Geometry: final body of the model. Coordinates: model frame, mm. A direction names the side the tool comes from. Round coordinates to 2 decimals unless told otherwise and drop trailing zeros. Loops run counter-clockwise (first coordinate to the right, second up) from the corner with the lowest first, then second, coordinate; pieces in that order, holes last. Notation, with made-up numbers: (49.25, 33.25) -> (102.25, 33.25) arc R21 ccw to (102.25, 67.25) -> close; hole circle Ø2 at (56, 63). An arc over 180 degrees is marked (long way). Answer in a Markdown table with one row per item.
```python
from build123d import *

# Parameters (mm, degrees)
SKETCH1_W               = 3.96875
SKETCH1_H               = 3.96875
BOSS_EXTRUDE1_DEPTH     = 12.5
SKETCH2_W               = 3.175
SKETCH2_H               = 3.175
CUT_EXTRUDE1_DEPTH      = 26.157016681
CUT_EXTRUDE2_DEPTH      = 13.811147032
CUT_EXTRUDE2_DEPTH_BACK = 13.811147032
SKETCH3_R               = 0.79375


with BuildPart() as part:
    # Sketch1 → Boss-Extrude1 (new, symmetric)
    with BuildSketch(Plane(origin=(0, 0, 0), x_dir=(1, 0, 0), z_dir=(0, 1, 0))):
        Rectangle(SKETCH1_W, SKETCH1_H)
    extrude(amount=BOSS_EXTRUDE1_DEPTH, both=True)

    # Sketch2 → Cut-Extrude1 (cut, through all)
    with BuildSketch(Plane(origin=(0, 12.5, 0), x_dir=(1, 0, 0), z_dir=(0, 1, 0))):
        Rectangle(SKETCH2_W, SKETCH2_H)
    extrude(amount=-CUT_EXTRUDE1_DEPTH, mode=Mode.SUBTRACT)

    # Sketch3 → Cut-Extrude2 (cut, two sides: drawn at the far end of the back side and taken through both)
    with BuildSketch(Plane.XY.offset(-CUT_EXTRUDE2_DEPTH_BACK)):
        with Locations((0, -10)):
            Circle(SKETCH3_R)
    extrude(amount=CUT_EXTRUDE2_DEPTH + CUT_EXTRUDE2_DEPTH_BACK, mode=Mode.SUBTRACT)


solid = part.part
```
Item 1: Cut plane A-A (x = 0). Output: boundary loops of the cut face in (y, z), then the cut area to 3 significant figures.
Answer:
| item | result |
|---|---|
| outline | (-12.5, -1.98) -> (-10.79, -1.98) -> (-10.79, -1.59) -> (-12.5, -1.59) -> close; (-12.5, 1.59) -> (-10.79, 1.59) -> (-10.79, 1.98) -> (-12.5, 1.98) -> close; (-9.21, -1.98) -> (12.5, -1.98) -> (12.5, -1.59) -> (-9.21, -1.59) -> close; (-9.21, 1.59) -> (12.5, 1.59) -> (12.5, 1.98) -> (-9.21, 1.98) -> close |
| area | 18.6 mm² |
Item 2: Reachability of faces 4 (the face through (-1.984, 0, 0)), 5 (the face through (0, 0, -1.588)) from +Z, -Z, +X, -X, +Y, -Y: full face, straight path, thin tool, end or side. Return the list, or none.
Answer:
| item | result |
|---|---|
| face 4 | +Z, -Z, -X, +Y, -Y |
| face 5 | +Y, -Y |
Item 3: Cut plane D-D (y = -10). Output: boundary loops of the cut face in (x, z).
Answer:
| item | result |
|---|---|
| outline | (-1.98, -1.98) -> (-0.79, -1.98) -> (-0.79, -1.59) -> (-1.59, -1.59) -> (-1.59, 1.59) -> (-0.79, 1.59) -> (-0.79, 1.98) -> (-1.98, 1.98) -> close; (0.79, -1.98) -> (1.98, -1.98) -> (1.98, 1.98) -> (0.79, 1.98) -> (0.79, 1.59) -> (1.59, 1.59) -> (1.59, -1.59) -> (0.79, -1.59) -> close |
Item 4: Cut plane C-C (z = 0.95). Output: boundary loops of the cut face in (x, y), then the cut area to 3 significant figures.
Answer:
| item | result |
|---|---|
| outline | (-1.98, -12.5) -> (-1.59, -12.5) -> (-1.59, 12.5) -> (-1.98, 12.5) -> close; (1.59, -12.5) -> (1.98, -12.5) -> (1.98, 12.5) -> (1.59, 12.5) -> close |
| area | 19.8 mm² |
Item 5: Line query: probe 1 along X at (y, z) = (0, -1.35); probe 2 along X at (y, z) = (-10, -1.8). Output: solid intervals per line, ascending. Write a range as [from, to].
Answer:
| item | result |
|---|---|
| probe 1 | x = [-1.98, -1.59], [1.59, 1.98] |
| probe 2 | x = [-1.98, -0.79], [0.79, 1.98] |
Item 6: Cut plane B-B (y = -2.25). Output: boundary loops of the cut face in (x, z).
Answer:
| item | result |
|---|---|
| outline | (-1.98, -1.98) -> (1.98, -1.98) -> (1.98, 1.98) -> (-1.98, 1.98) -> close; hole (-1.59, -1.59) -> (1.59, -1.59) -> (1.59, 1.59) -> (-1.59, 1.59) -> close |
Item 7: Draft query along X for faces 1 (the face through (-0.172, -10.775, 1.783)), 2 (the face through (1.984, 0, 0)), 3 (the face through (-1.8, 12.5, 0)). Return one class per face: pulls with the +X half, pulls with the -X half, needs draft (parallel to the pull), parting line crosses it, or undercut.
Answer:
| item | result |
|---|---|
| face 1 | undercut |
| face 2 | pulls with the +X half |
| face 3 | needs draft |
